Check sheet for the modelled part. Datum: model origin and axes. Units: mm. A direction names the side the tool comes from. Give positions to 0.01 mm unless a question says otherwise; leave off trailing zeros. Loops run counter-clockwise (first coordinate to the right, second up) from the corner with the lowest first, then second, coordinate; pieces in that order, holes last. Notation, with made-up numbers: (8, 19) -> (38, 19) arc R11 ccw to (38, 38) -> close; hole circle Ø10 at (23, -17.75). An arc over 180 degrees is marked (long way). Answer as CSV lines item,"result". Start each with the question number.
(1) Section check C-C on y = -1. Enter the section's corners in (x, z).
(2) Gauge pin test, flat ends, axial feed: pin 1 Ø4 at (y, z) = (35.5, 22) entering from -X; pin 2 Ø6 at (x, z) = (22, 10.5) entering from -Y; pin 3 Ø10 at (y, z) = (11, 2.5) entering from +X; pin 4 Ø23.5 at (x, y) = (-11, 4) entering from +Z. Record the tip position at first contact, or that the pin passes through.
(3) Material ranges on line 1 (Y direction, x = 13.5, z = 16.25); line 2 (Y direction, x = -32.5, z = 9.25); line 3 (Y direction, x = 27.5, z = 6.5), recorded low to high. Write a range as from..to.
(4) Section check B-B on x = -25.5. Enter the section's corners in (y, z).
(5) Section check D-D on x = 14. Enter the section's corners in (y, z), plus the area to 3 significant figures.
(6) Section check A-A on z = 4.5. Enter the section's corners in (x, y).
(7) Release check for a two-part mould opening along X. For faces 1 (the face through (8.05, 44.62, 12.52)), 2 (the face through (12.478, 3.004, 12.522)), 3 (the face through (-6, -3, 0)), 4 (the face through (18.415, 44.709, 13.166)) record: pulls with the +X half, pulls with the -X half, needs draft (parallel to the pull), parting line crosses it, or undercut.
(8) Access from +Z, -Z, +X, -X, +Y, -Y to the whole of each face (thin tool, end or side, straight path). Record for faces 5 (the face through (-7, 19.757, 13)), 6 (the face through (2, -22.279, 13)), 7 (the face through (9.919, 1.734, 13.166)).
from build123d import *

# Parameters (mm, degrees)
F1_DEPTH = 25.4
F2_T     = -1.27


with BuildPart() as f1:
    # F0 (on Top) → F1 (new body)
    with BuildSketch(Plane.XY):
        Polygon((11.7702977732, 29.0053766221), (32.2281979024, 68.8001960516), (-16.8147105724, 19.7572857141), (3.0826970469, 19.7572857141), (-41.1960408092, -30.406601727), (-20.7381434739, -30.406601727), (-57.4502646923, -76.0865658522), (9.7388841726, -22.2794916481), (-6.7258845083, -22.2794916481), (32.2281979024, 29.0053766221), align=None)
    extrude(amount=F1_DEPTH)

    # F2
    f2_openings = [f1.faces().sort_by_distance(p)[0] for p in [
        (-5.320253, -2.614371, 25.4),
    ]]
    offset(amount=F2_T, openings=f2_openings, kind=Kind.INTERSECTION)


solid = f1.part
Working result:
1,outline,"(-15.24, 0) -> (9.44, 0) -> (9.44, 25.4) -> (7.84, 25.4) -> (7.84, 1.27) -> (-13.55, 1.27) -> (-13.55, 25.4) -> (-15.24, 25.4) -> close"
2,pin 1,"stops at x = -3.07"
2,pin 2,"stops at y = 11.59"
2,pin 3,"stops at x = 22.35"
2,pin 4,"stops at z = 25.4"
3,line 1,"y = 4.35..6.45, 27.74..29.01, 32.37..35.15, 48.28..50.07"
3,line 2,"y = -56.11..-54.48, -47.07..-45.04, -30.41..-29.14, -22.47..-20.55"
3,line 3,"y = 22.78..24.88, 27.74..29.01, 59.6..64.07"
4,outline,"(-50.5, 0) -> (-36.33, 0) -> (-36.33, 25.4) -> (-38.36, 25.4) -> (-38.36, 1.27) -> (-48.87, 1.27) -> (-48.87, 25.4) -> (-50.5, 25.4) -> close; (-30.41, 0) -> (-12.62, 0) -> (-12.62, 25.4) -> (-14.54, 25.4) -> (-14.54, 1.27) -> (-29.14, 1.27) -> (-29.14, 25.4) -> (-30.41, 25.4) -> close"
5,outline,"(5.01, 0) -> (29.01, 0) -> (29.01, 25.4) -> (27.74, 25.4) -> (27.74, 1.27) -> (7.11, 1.27) -> (7.11, 25.4) -> (5.01, 25.4) -> close; (33.34, 0) -> (50.57, 0) -> (50.57, 25.4) -> (48.78, 25.4) -> (48.78, 1.27) -> (36.12, 1.27) -> (36.12, 25.4) -> (33.34, 25.4) -> close"
5,area,"244 mm^2"
6,outline,"(-57.45, -76.09) -> (9.74, -22.28) -> (-6.73, -22.28) -> (32.23, 29.01) -> (11.77, 29.01) -> (32.23, 68.8) -> (-16.81, 19.76) -> (3.08, 19.76) -> (-41.2, -30.41) -> (-20.74, -30.41) -> close; hole (-49.21, -67.86) -> (6.12, -23.55) -> (-9.29, -23.55) -> (29.67, 27.74) -> (9.69, 27.74) -> (27.39, 62.17) -> (-13.75, 21.03) -> (5.9, 21.03) -> (-38.38, -29.14) -> (-18.09, -29.14) -> close"
7,face 1,"pulls with the -X half"
7,face 2,"pulls with the +X half"
7,face 3,"needs draft"
7,face 4,"undercut"
8,face 5,"+Z, -Z, -X"
8,face 6,"+Z, -Z, +X"
8,face 7,"+Z"
